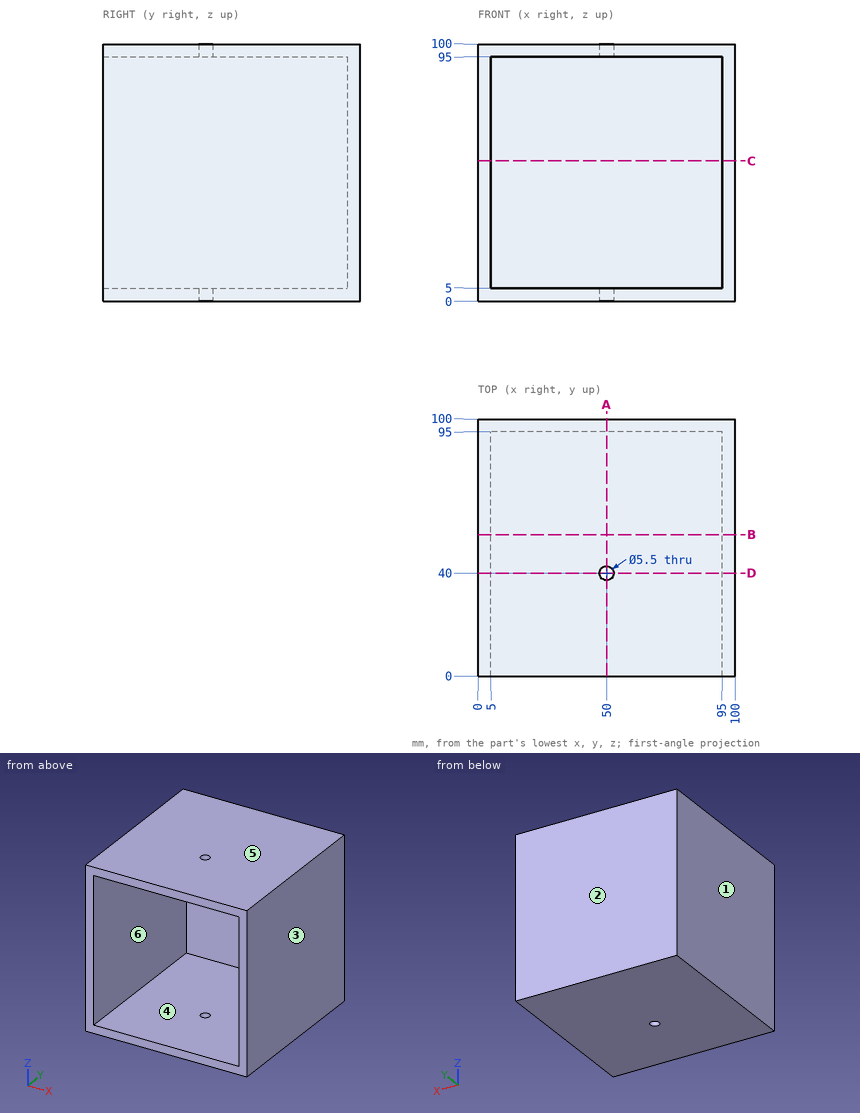
Geometry check sheet. Reference: drawing and pictorial views, mm from the part's lowest x, y, z. A direction names the side the tool comes from. Round coordinates to 2 decimals unless told otherwise and drop trailing zeros. Loops run counter-clockwise (first coordinate to the right, second up) from the corner with the lowest first, then second, coordinate; pieces in that order, holes last.
1. Sectioned sample at A-A on x = 50. Record the boundary of the cut face in (y, z).
2. Scan lines: probe 1 along Z at (x, y) = (41, 35); probe 2 along Y at (x, z) = (50, 1.95). Record each from-to range of solid material in increasing order.
3. Mould release check, pull along X, two halves, no side actions. Record for the marked faces 1, 2, 3 and 4: released by +X, released by -X, zero draft, split by the parting line, or undercut.
4. Sectioned sample at C-C on z = 54.5. Record the boundary of the cut face in (x, y), and give its area (3 significant figures).
5. Sectioned sample at B-B on y = 55. Record the boundary of the cut face in (x, z), and give its area (3 significant figures).
6. Set-up check for the marked faces 5 and 6: record each of +Z, -Z, +X, -X, +Y, -Y from which the full face is reachable in a straight line by a thin tool's end or side.
7. Sectioned sample at D-D on y = 40. Record the boundary of the cut face in (x, z).
8. Gauge pin test, flat end, axial feed: pin 1 Ø2 at (x, z) = (58, 87.5) entering from -Y. Record the tip position at first contact, or that the pin passes through.
Recorded:
1. outline: (0, 0) - (37.25, 0) - (37.25, 5) - (0, 5) - close; (0, 95) - (37.25, 95) - (37.25, 100) - (0, 100) - close; (42.75, 0) - (100, 0) - (100, 100) - (42.75, 100) - (42.75, 95) - (95, 95) - (95, 5) - (42.75, 5) - close
2. probe 1: z = 0 to 5, 95 to 100
2. probe 2: y = 0 to 37.25, 42.75 to 100
3. face 1: released by -X
3. face 2: zero draft
3. face 3: released by +X
3. face 4: undercut
4. outline: (0, 0) - (5, 0) - (5, 95) - (95, 95) - (95, 0) - (100, 0) - (100, 100) - (0, 100) - close
4. area: 1,450 mm2
5. outline: (0, 0) - (100, 0) - (100, 100) - (0, 100) - close; hole (5, 5) - (95, 5) - (95, 95) - (5, 95) - close
5. area: 1,900 mm2
6. face 5: +Z, +X, -X, +Y, -Y
6. face 6: -Y
7. outline: (0, 0) - (47.25, 0) - (47.25, 5) - (5, 5) - (5, 95) - (47.25, 95) - (47.25, 100) - (0, 100) - close; (52.75, 0) - (100, 0) - (100, 100) - (52.75, 100) - (52.75, 95) - (95, 95) - (95, 5) - (52.75, 5) - close
8. pin 1: stops at y = 95
